The listing builds one solid part. Answer for the finished solid, in the listing's coordinates (mm). Face numbers are marked on the shaded views. A direction names the side the tool comes from. Coordinates: 2 decimals unless noted, no trailing zeros. Loops run counter-clockwise (first coordinate to the right, second up) from the corner with the lowest first, then second, coordinate; pieces in that order, holes last. Notation, with made-up numbers: (31, 88.5) - (69, 88.5) arc R7 cw to (69, 96.5) - close; hole circle Ø2 at (88.25, 67). An arc over 180 degrees is marked (long way). Put each result on its own line as item: value.
Autodesk Inventor part; units mm, degrees
ref_plane "YZ Plane" through (0, 0, 0) normal (1, 0, 0) x (0, 1, 0)
ref_plane "XZ Plane" through (0, 0, 0) normal (0, 1, 0) x (-1, 0, 0)
ref_plane "XY Plane" through (0, 0, 0) normal (0, 0, 1) x (1, 0, 0)
sketch "Sketch1" plane through (0, 0, 0) normal (0, 1, 0) x (-1, 0, 0)
  line L0 (-13.75, 3.5) -> (13.75, 3.5)
  line L1 (13.75, 3.5) -> (13.75, -3.5)
  line L2 (13.75, -3.5) -> (-13.75, -3.5)
  line L3 (-13.75, -3.5) -> (-13.75, 3.5)
  line L4 (-13.75, 3.5) -> (13.75, -3.5) construction
  line L5 (13.75, 3.5) -> (-13.75, -3.5) construction
  point P0 (0, 0)
  dimension "d0" = 27.5
  dimension "d1" = 7
extrude "Extrusion1" add sketch "Sketch1" along normal blind 2.5
sketch "Sketch2" plane through (13.75, 0, -3.5) normal (0, 0, -1) x (-1, 0, 0)
  line L0 (27.5, 0) -> (27.5, 2.5)
  line L1 (27.5, 1.25) -> (26, 1.25)
  circle A0 centre (26, 1.25) radius 1
  point P0 (13.75, 0)
  dimension "d4" = 1.5
  dimension "d5" = 2
extrude "Extrusion2" add sketch "Sketch2" along normal blind 2 draft -12
sketch "Sketch3" plane through (13.75, 0, 3.5) normal (1, 0, 0) x (0, 0, -1)
  line L0 (0, 2.5) -> (7, 2.5)
  line L1 (3.5, 2.5) -> (3.5, -12.5)
  line L2 (7, 0) -> (7, 2.5)
  arc A0 (14.3915, -1.6085) -> (7, 2.5) centre (3.5, -12.5) ccw
  arc A1 (12.6788, -3.3212) -> (3.5, 0.4808) centre (3.5, -12.5) ccw
  line L3 (3.5, -12.5) -> (14.3915, -1.6085)
  line L4 (3.5, -12.5) -> (18.9029, -12.5) construction
  line L5 (7, 0) -> (7, 2.5)
  point P0 (3.5, 0)
  dimension "d8" = 15
  dimension "d9" = 45
extrude "Extrusion3" add sketch "Sketch3" against normal blind 12 contours L0 L2 A1 L1 | A0 L3 A1 L2
sketch "Sketch4" plane through (-13.75, 0, 3.5) normal (0, 0, 1) x (1, 0, 0)
  line L0 (0, 2.5) -> (27.5, 2.5)
  line L1 (13.75, 2.5) -> (15.75, 2.5)
  line L2 (15.75, 2.5) -> (11.75, 2.5)
  line L3 (11.75, 2.5) -> (11.75, 3.5)
  line L4 (11.75, 3.5) -> (15.75, 3.5)
  line L5 (15.75, 3.5) -> (15.75, 2.5)
  arc A0 (11.75, 3.5) -> (15.75, 3.5) centre (13.75, 5) ccw
  point P0 (13.75, 0)
  dimension "d12" = 2
  dimension "d13" = 4
  dimension "d14" = 1
extrude "Extrusion4" add sketch "Sketch4" against normal blind 3.5 contours L3 A0 L0 | A0 L5 L0
fillet "Fillet1" radius 4 1 edges at (1.75, 1.25, -3.5)
mirror "Mirror1" about plane through (1.2398, 2.7314, 0) normal (0, 0, -1)
ref_plane "Work Plane1" through (2, 2.5, 9.5) normal (0, 0, 1) x (1, 0, 0)
sketch "Sketch6" plane through (2, 2.5, 9.5) normal (0, 0, 1) x (1, 0, 0)
  line L0 (11.75, -2.5) -> (11.75, -5.8212)
  line L1 (11.75, -5.8894) -> (11.75, -2.5)
  line L2 (-4.25, -2.5) -> (11.75, -2.5)
  line L3 (11.75, -2.5) -> (-0.25, -2.5)
  arc A0 (11.75, -5.8212) -> (-0.25, -2.5) centre (-2.078, -32.4443) ccw
  point P0 (-2, -2.5)
  dimension "d25" = 12
  dimension "d26" = 30
extrude "Extrusion6" add sketch "Sketch6" against normal blind 19
properties part number "index_clamp"
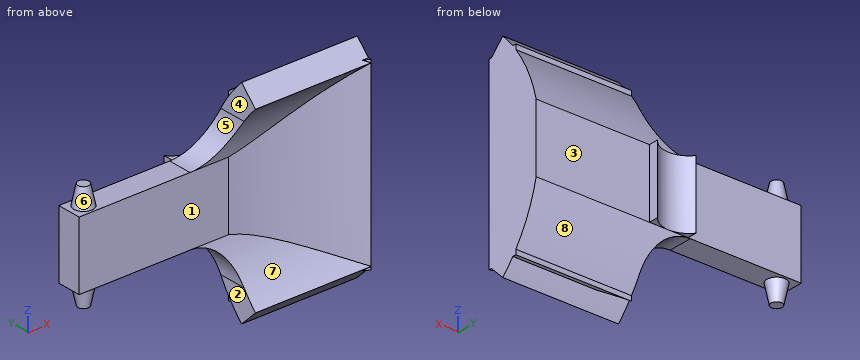
1) The part is cut by section D-D (z = 5). Give the vertices of the cut face in (x, y).
Found:
outline: circle Ø1.36 at (-12.25, 1.25); (0.87, -0.52) - (5.78, -0.52) arc R30 cw to (13.75, -3.32) - (13.75, 2.07) - (0.87, 2.07) - close
2) For a pull along Z with two mould halves and no side action, classify the marked faces 6, 7 and 8 as pulls with the +Z half, pulls with the -Z half, needs draft (parallel to the pull), parting line crosses it, or undercut.
Found:
face 6: pulls with the +Z half
face 7: undercut
face 8: pulls with the -Z half
3) The part is cut by section A-A (z = 2.5). Give the vertices of the cut face in (x, y), and give its area (3 significant figures).
Found:
outline: (-13.75, 0) - (1.75, 0) arc R30 cw to (13.75, -3.32) - (13.75, 2.5) - (2, 2.5) - (2, 3.5) arc R2.5 cw to (-2, 3.5) - (-2, 2.5) - (-13.75, 2.5) - close
area: 84.4 mm^2
4) Straight lines are drawn through the part: L1, parallel to Y at x = -10.5, z = 2.5; L2, parallel to Y at x = 5.5, z = 7.5; L3, parallel to Z at x = -6, y = 0.5. For each, find the intervals that lie inside material, in ascending order. Write a range as [from, to].
Found:
L1: y = [0, 2.5]
L2: y = [-1.91, 0.95]
L3: z = [-3.5, 3.5]
5) The part is cut by section C-C (y = -1). Give the vertices of the cut face in (x, z), and give its area (3 significant figures).
Found:
outline: (1.47, -6.02) arc R4 cw to (1.75, -7.5) - (1.75, -10.25) - (13.75, -10.25) - (13.75, 10.25) - (1.75, 10.25) - (1.75, 7.5) arc R4 cw to (1.47, 6.02) - (7.81, 6.02) - (7.81, -6.02) - close
area: 173 mm^2
6) Each of these flat-tipped pins is pushed along its axis until it touches: pin 1 (7.5 mm diameter, centred on x = -10.5, z = -0.5, fed in from +Y); pin 2 (1.2 mm diameter, centred on x = -5.5, y = 1, fed in from +Z); pin 3 (4 mm diameter, centred on x = 5, z = 6.5, fed in from +Y). Where does it stop, or does it pass through?
Found:
pin 1: stops at y = 2.5
pin 2: stops at z = 3.5
pin 3: stops at y = 2.23
7) For the marked faces 1, 2, 3, 4 and 5, determine the directions among +Z, -Z, +X, -X, +Y, -Y from which every point of the face is accessible in a straight line to the end or side of a thin tool.
Found:
face 1: -X, -Y
face 2: -Z, -X, +Y, -Y
face 3: +Z, -Z, +X, +Y
face 4: +Z, -X, +Y, -Y
face 5: +Z, +Y, -Y
8) The part is cut by section B-B (x = -12.25). Give the vertices of the cut face in (y, z).
Found:
outline: (0, -3.5) - (0.25, -3.5) - (0.68, -5.5) - (1.82, -5.5) - (2.25, -3.5) - (2.5, -3.5) - (2.5, 3.5) - (2.25, 3.5) - (1.82, 5.5) - (0.68, 5.5) - (0.25, 3.5) - (0, 3.5) - close
